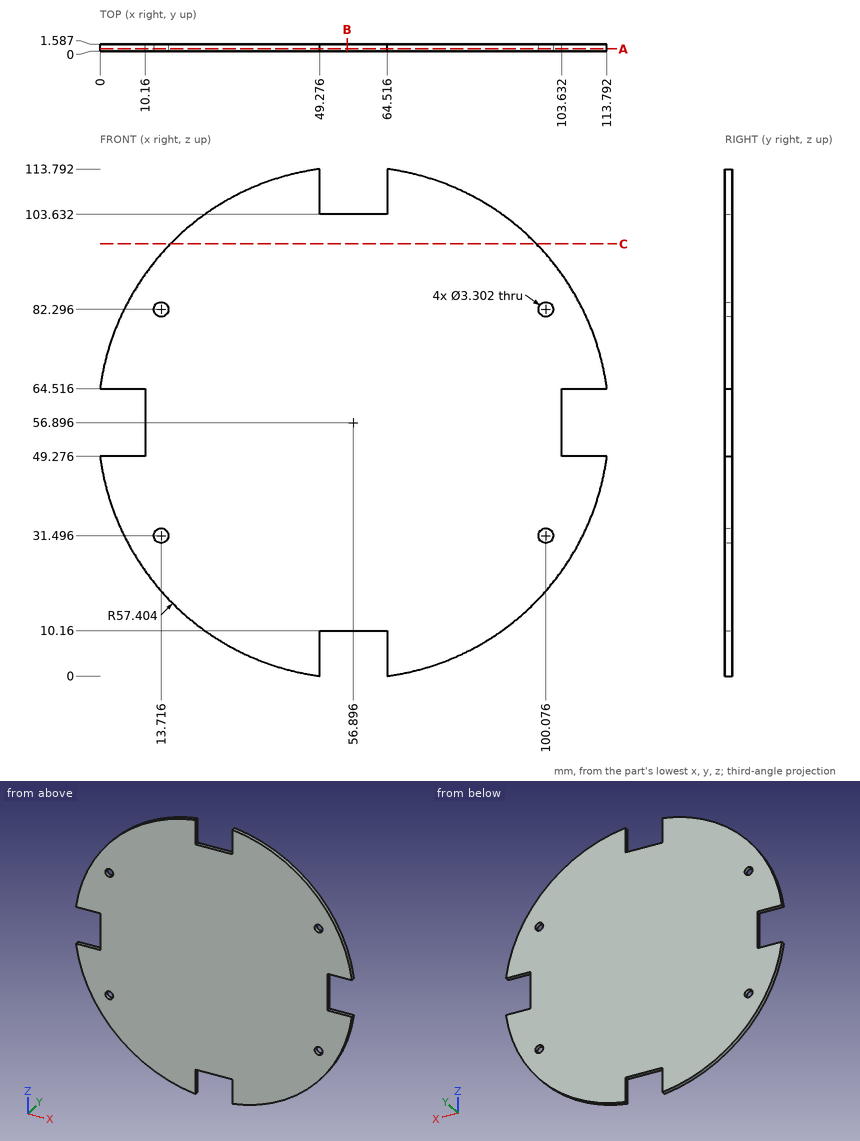
The figure shows three views and two pictorial views of one solid part (mm, origin at its lowest corner). Answer the questions. Round coordinates to 2 decimals unless told otherwise and drop trailing zeros. Write each loop counter-clockwise with the first axis right and the second up, starting at its lowest first coordinate (ties: lowest second). Pieces come first, ordered by that corner, then holes. Notation, with made-up numbers: (-12.75, 62.5) -> (18.25, 62.5) arc R26 ccw to (18.25, 100.5) -> close; hole circle Ø2 at (38.5, 26). An arc over 180 degrees is marked (long way). Answer as a JSON object with one key per item and string values. Group by question number.
Q1. Straight lines are drawn through the part: line 1 along Z through (x, y) = (52, 0.95); line 2 along X through (y, z) = (0.7, 107) (1 decimal). For each, find the intervals that lie inside material, in ascending order.
Q2. Each of these flat-tipped pins is pushed along its axis until it touches: pin 1 Ø0.8 at (x, y) = (59, 1) entering from +Z; pin 2 Ø0.8 at (x, y) = (6.5, 1) entering from +Z (1 decimal); pin 3 Ø3 at (x, z) = (13.716, 31.496) entering from -Y; pin 4 Ø0.8 at (y, z) = (1, 110.5) entering from +X. Where does it stop, or does it pass through?
Q3. Section B-B (x = 55.5) is taken. Write down the section's boundary in (y, z).
Q4. Section C-C (z = 97) is taken. Write down the section's boundary in (x, y) (1 decimal).
Q5. Section A-A (y = 0.5) is taken. Count the separate pieces of the cut face and the enclosed holes in it, plus the area to 3 significant figures.
Check values:
{
 "1": {"line 1": "10.16 to 103.63", "line 2": "28.9 to 49.3, 64.5 to 84.9"},
 "2": {"pin 1": "z = 103.63", "pin 2": "z = 85.1", "pin 3": "through", "pin 4": "x = 78.45"},
 "3": {"outline": "(0, 10.16) -> (1.59, 10.16) -> (1.59, 103.63) -> (0, 103.63) -> close"},
 "4": {"outline": "(15.8, 0) -> (98, 0) -> (98, 1.6) -> (15.8, 1.6) -> close"},
 "5": {"separate pieces": "1", "enclosed holes": "4", "area": "9,680 mm^2"}
}
